Read the model definition and answer for the solid it produces. Units are mm, in the model's axes. Round coordinates to 2 decimals unless told otherwise and drop trailing zeros. Loops run counter-clockwise (first coordinate to the right, second up) from the corner with the lowest first, then second, coordinate; pieces in that order, holes last. Notation, with made-up numbers: (-35.75, 12.5) - (-18.75, 12.5) arc R25 ccw to (-18.75, 50.5) - close; hole circle Ø9 at (-9, -25). An arc over 180 degrees is marked (long way). Use one line per item in the form item = value. Start each with the question number.
Autodesk Inventor part; units mm, degrees
ref_plane "YZ Plane" through (0, 0, 0) normal (1, 0, 0) x (0, 1, 0)
ref_plane "XZ Plane" through (0, 0, 0) normal (0, 1, 0) x (-1, 0, 0)
ref_plane "XY Plane" through (0, 0, 0) normal (0, 0, 1) x (1, 0, 0)
sketch "Sketch1" plane through (0, 0, 0) normal (0, 0, 1) x (1, 0, 0)
  circle A0 centre (0, 0) radius 16
  circle A1 centre (0, 0) radius 6
  dimension "d0" = 32
  dimension "d1" = 12
extrude "Extrusion1" add sketch "Sketch1" along normal blind 10
fillet "Fillet1" radius 2 2 edges at (-16, 0, 10) (-16, 0, 0)
fillet "Fillet2" radius 1 2 edges at (-6, 0, 10) (-6, 0, 0)
properties part number "6201RS" material "Steel, Carbon"
1) A cutting plane is placed at C-C on z = 6.25. Write down the section's boundary in (x, y).
2) Flat-ended cylindrical pins translate along their axes: pin 1 (1.5 mm diameter, centred on y = -7, z = 2.5, fed in from -X); pin 2 (4 mm diameter, centred on x = -7, z = 3, fed in from +Y); pin 3 (3 mm diameter, centred on x = 9, z = 5, fed in from +Y). Find the tip coordinate at first contact, or state that the pin passes through.
3) A cutting plane is placed at A-A on y = 0. Write down the section's boundary in (x, z).
4) Determine the mould class of faces 1 (the cylindrical face through (-3.47, 15.62, 4.96)), 2 (the flat face through (-6.4, 3.3, 10)), 3 (the cylindrical face through (-6, 0, 5)) for opening direction Y: +Y half, -Y half, draft (parallel to the pull), parting line (faces both ways), or undercut.
5) Straight lines are drawn through the part: line 1 (X direction, y = -3, z = 4); line 2 (Z direction, x = 7.5, y = 12); line 3 (Y direction, x = 1.5, z = 3.5). For each, find the intervals that lie inside material, in ascending order. Write a range as from..to.
Checks:
q1.outline = circle Ø32 at (0, 0); hole circle Ø12 at (0, 0)
q2.pin_1 = -14.73
q2.pin_2 = 15.2
q2.pin_3 = 14.13
q3.outline = (-16, 2) arc R2 ccw to (-14, 0) - (-7, 0) arc R1 ccw to (-6, 1) - (-6, 9) arc R1 ccw to (-7, 10) - (-14, 10) arc R2 ccw to (-16, 8) - close; (6, 1) arc R1 ccw to (7, 0) - (14, 0) arc R2 ccw to (16, 2) - (16, 8) arc R2 ccw to (14, 10) - (7, 10) arc R1 ccw to (6, 9) - close
q4.face_1 = parting line
q4.face_2 = draft
q4.face_3 = undercut
q5.line_1 = -15.72..-5.2, 5.2..15.72
q5.line_2 = 0.01..9.99
q5.line_3 = -15.93..-5.81, 5.81..15.93
